Check sheet for the modelled part. Datum: model origin and axes. Units: mm. A direction names the side the tool comes from. Coordinates: 2 decimals unless noted, no trailing zeros. Loops run counter-clockwise (first coordinate to the right, second up) from the corner with the lowest first, then second, coordinate; pieces in that order, holes last.
from build123d import *

# Parameters (mm, degrees)
F1_DEPTH = 12.5


with BuildPart() as f1:
    # F0 (on Front) → F1 (new body, symmetric)
    with BuildSketch(Plane.XZ):
        with BuildLine():
            Line((0, 4.5), (0, 0))
            Line((0, 0), (76.2, 0))
            Line((76.2, 0), (76.2, 4.5))
            Line((76.2, 4.5), (43.322799, 4.5))
            ThreePointArc((43.322799, 4.5), (42.322799, 4.767949), (41.590748, 5.5))
            Line((41.590748, 5.5), (41.1, 6.35))
            ThreePointArc((41.1, 6.35), (38.1, 3.35), (35.1, 6.35))
            Line((35.1, 6.35), (34.609252, 5.5))
            ThreePointArc((34.609252, 5.5), (33.877201, 4.767949), (32.877201, 4.5))
            Line((32.877201, 4.5), (0, 4.5))
        make_face()
    extrude(amount=F1_DEPTH, both=True)


solid = f1.part
(1) Draft check along X on faces 3 (the face through (38.17, -0.18, 3.35)), 4 (the face through (0, 0, 2)), 5 (the face through (17, 0, 4.5)). Enter one of: pulls with the +X half, pulls with the -X half, needs draft (parallel to the pull), parting line crosses it, or undercut.
(2) Gauge pin test, flat ends, axial feed: P1, Ø5, axis at x = 27.5, y = -2.5, coming from the +Z side; P2, Ø1, axis at x = 63.5, z = 5.5, coming from the +Y side. Record the tip position at first contact, or that the pin passes through.
(3) Scan lines: line 1 along Z through (x, y) = (4, 7.75); line 2 along X through (y, z) = (10.25, 4.25); line 3 along X through (y, z) = (2, 5.25). Record each from-to range of solid material in increasing order.
(4) Section check C-C, the plane x = 24. Enter the section's corners in (y, z).
(5) Set-up check for faces 1 (the face through (38, -12.5, 2)), 2 (the face through (60, 0, 4.5)): record each of +Z, -Z, +X, -X, +Y, -Y from which the full face is reachable in a straight line by a thin tool's end or side.
(6) Section check B-B, the plane x = 38.1. Enter the section's corners in (y, z), plus the area to 4 significant figures.
(7) Section check A-A, the plane y = -9. Enter the section's corners in (x, z), plus the area to 3 significant figures.
Determined:
1. face 3: undercut
1. face 4: pulls with the -X half
1. face 5: needs draft
2. P1: stops at z = 4.5
2. P2: passes through
3. line 1: z = 0 to 4.5
3. line 2: x = 0 to 35.96, 40.24 to 76.2
3. line 3: x = 34.44 to 35.31, 40.89 to 41.76
4. outline: (-12.5, 0) - (12.5, 0) - (12.5, 4.5) - (-12.5, 4.5) - close
5. face 1: +Z, -Z, +X, -X, -Y
5. face 2: +Z, +X, +Y, -Y
6. outline: (-12.5, 0) - (12.5, 0) - (12.5, 3.35) - (-12.5, 3.35) - close
6. area: 83.75 mm2
7. outline: (0, 0) - (76.2, 0) - (76.2, 4.5) - (43.32, 4.5) arc R2 cw to (41.59, 5.5) - (41.1, 6.35) arc R3 cw to (35.1, 6.35) - (34.61, 5.5) arc R2 cw to (32.88, 4.5) - (0, 4.5) - close
7. area: 342 mm2
